Autodesk Inventor part; units mm, degrees
ref_plane "YZ Plane" through (0, 0, 0) normal (1, 0, 0) x (0, 1, 0)
ref_plane "XZ Plane" through (0, 0, 0) normal (0, 1, 0) x (-1, 0, 0)
ref_plane "XY Plane" through (0, 0, 0) normal (0, 0, 1) x (1, 0, 0)
sketch "Sketch1" plane through (0, 0, 0) normal (0, 1, 0) x (-1, 0, 0)
  line L0 (-88.0953, -35.095) -> (-78.6953, -35.095)
  line L1 (62.5047, 52.705) -> (71.9047, 52.705)
  line L2 (-88.0953, -35.095) -> (71.9047, -35.095)
  line L3 (71.9047, -35.095) -> (71.9047, 52.705)
  line L4 (71.9047, 52.705) -> (-88.0953, 52.705)
  line L5 (-88.0953, 52.705) -> (-88.0953, -35.095)
  circle A0 centre (-79.9551, -5.92) radius 2.7
  circle A1 centre (-79.9551, -5.92) radius 2.7
  circle A2 centre (-79.9551, 23.53) radius 2.7
  circle A3 centre (-79.9551, 23.53) radius 2.7
  circle A4 centre (-8.0953, 8.805) radius 2.7
  circle A5 centre (-8.0953, 8.805) radius 2.7
  circle A6 centre (63.7645, -5.92) radius 2.7
  circle A7 centre (63.7645, -5.92) radius 2.7
  circle A8 centre (63.7645, 23.53) radius 2.7
  circle A9 centre (63.7645, 23.53) radius 2.7
  line L6 (-88.0953, -35.095) -> (71.9047, -35.095)
  line L7 (71.9047, -35.095) -> (71.9047, 52.705)
  line L8 (71.9047, 52.705) -> (-88.0953, 52.705)
  line L9 (-88.0953, 52.705) -> (-88.0953, -35.095)
  point P0 (0, 0)
  point P1 (-83.0953, -33.095)
extrude "Extrusion1" add sketch "Sketch1" along normal blind 3
sketch "Sketch2" plane through (0, 3, 0) normal (0, 1, 0) x (1, 0, 0)
  circle A0 centre (8.0953, -8.805) radius 2.7
  line L0 (8.0953, -8.805) -> (8.0953, -52.705)
  line L1 (-71.9047, -52.705) -> (88.0953, -52.705)
  line L2 (8.0953, -8.805) -> (8.0953, 35.095)
  line L3 (88.0953, 35.095) -> (-71.9047, 35.095)
  line L4 (8.0953, -8.805) -> (-35.8047, -52.705)
  line L5 (8.0953, -8.805) -> (70.1793, -8.805) construction
  line L6 (8.0953, -8.805) -> (51.9953, -52.705)
  line L7 (8.0953, -8.805) -> (70.1793, -8.805) construction
  line L8 (8.0953, -8.805) -> (-18.3888, -8.805)
  line L9 (8.0953, -8.805) -> (-35.8047, 35.095)
  line L10 (8.0953, -8.805) -> (51.9953, 35.095)
  line L11 (-35.8047, -52.705) -> (51.9953, -52.705)
  line L12 (51.9953, -52.705) -> (51.9953, 35.095)
  line L13 (51.9953, 35.095) -> (-35.8047, 35.095)
  line L14 (-35.8047, 35.095) -> (-35.8047, -52.705)
  line L15 (8.0953, -8.805) -> (8.0953, -28.805)
  line L16 (8.0953, -28.805) -> (8.0953, 11.195)
  line L17 (8.0953, 11.195) -> (-15.8047, 35.095)
  line L18 (8.0953, -28.805) -> (-15.8047, -52.705)
  line L19 (8.0953, -28.805) -> (31.9953, -52.705)
  line L20 (8.0953, 11.195) -> (31.9953, 35.095)
  point P0 (0, 0)
  dimension "d2" = 135
  dimension "d3" = 45
  dimension "d4" = 20
  dimension "d5" = 40
extrude "Extrusion2" cut sketch "Sketch2" against normal blind 3 contours L17 L3 L2 | L2 L3 L20 | L19 L1 L0 | L0 L1 L18
sketch "Sketch3" plane through (0, 3, 0) normal (0, 1, 0) x (1, 0, 0)
  line L0 (-71.9047, 35.095) -> (-71.9047, -52.705)
  line L1 (-71.9047, -8.805) -> (-34.7047, -8.805)
  circle A0 centre (-34.7047, -8.805) radius 10
  point P0 (0, 0)
  dimension "d8" = 37.2
  dimension "d9" = 20
extrude "Extrusion3" cut sketch "Sketch3" against normal blind 3
sketch "Sketch4" plane through (0, 3, 0) normal (0, 1, 0) x (1, 0, 0)
  point P0 (0, 0)
sketch "Sketch5" plane through (0, 3, 0) normal (0, 1, 0) x (1, 0, 0)
  line L0 (-71.9047, 35.095) -> (-71.9047, -52.705)
  line L1 (88.0953, -52.705) -> (88.0953, 35.095)
  line L2 (-71.9047, -52.705) -> (88.0953, -52.705)
  line L3 (8.0953, -52.705) -> (8.0953, 35.095)
  circle A0 centre (-34.7047, -8.805) radius 10
  circle A1 centre (-34.7047, -8.805) radius 10
  circle A2 centre (50.8953, -8.805) radius 10
  point P0 (0, 0)
extrude "Extrusion4" cut sketch "Sketch5" against normal blind 3 contours A2
sketch "Sketch6" plane through (0, 3, 0) normal (0, 1, 0) x (1, 0, 0)
  line L0 (-48.5025, 4.8798) -> (-18.5618, 4.8798)
  line L1 (-18.5618, 4.8798) -> (-18.5618, -20.2546)
  line L2 (-18.5618, -20.2546) -> (-48.5025, -20.2546)
  line L3 (-48.5025, -20.2546) -> (-48.5025, 4.8798)
  point P0 (0, 0)
extrude "Extrusion5" add sketch "Sketch6" against normal up to surface (3 mm away)
sketch "Sketch7" plane through (0, 3, 0) normal (0, 1, 0) x (1, 0, 0)
  line L0 (-15.8047, 35.095) -> (-71.9047, 35.095)
  line L1 (-71.9047, 35.095) -> (8.0953, 35.095)
  line L2 (8.0953, 35.095) -> (8.0953, -52.705)
  line L3 (8.0953, -52.705) -> (-71.9047, -52.705)
  line L4 (-71.9047, -52.705) -> (-71.9047, 35.095)
  line L5 (-71.9047, -8.805) -> (8.0953, -8.805)
  line L6 (-31.9047, -8.805) -> (-52.4047, -8.805)
  line L7 (-52.4047, -8.805) -> (-11.4047, -8.805)
  line L8 (-52.4047, -8.805) -> (-11.4047, -8.805)
  line L9 (-11.4047, -8.805) -> (-11.4047, 25.695)
  line L10 (-11.4047, 25.695) -> (-52.4047, 25.695)
  line L11 (-52.4047, 25.695) -> (-52.4047, -8.805)
  line L12 (-52.4047, 25.695) -> (-11.4047, 25.695)
  line L13 (-11.4047, 25.695) -> (-11.4047, -43.305)
  line L14 (-11.4047, -43.305) -> (-52.4047, -43.305)
  line L15 (-52.4047, -43.305) -> (-52.4047, 25.695)
  line L16 (-31.9047, -8.805) -> (-31.9047, -5.9886)
  line L17 (-31.9047, -5.9886) -> (-50.3547, -5.9886)
  line L18 (-50.3547, -5.9886) -> (-13.4547, -5.9886)
  line L19 (-50.4047, 23.695) -> (-13.4047, 23.695)
  line L20 (-13.4047, 23.695) -> (-13.4047, -41.305)
  line L21 (-13.4047, -41.305) -> (-50.4047, -41.305)
  line L22 (-50.4047, -41.305) -> (-50.4047, 23.695)
  point P0 (0, 0)
  dimension "d16" = 20.5
  dimension "d17" = 41
  dimension "d18" = 34.5
  dimension "d19" = 69
  dimension "d20" = 18.45
  dimension "d21" = 36.9
  dimension "d22" = 2
extrude "Extrusion6" add sketch "Sketch7" along normal blind 18.5 contours L11 L10 L9 L5 L20 L19 L22 | L5 L22 L21 L20 L13 L14 L15
properties part number "SCHOOL PROJECT TOP"
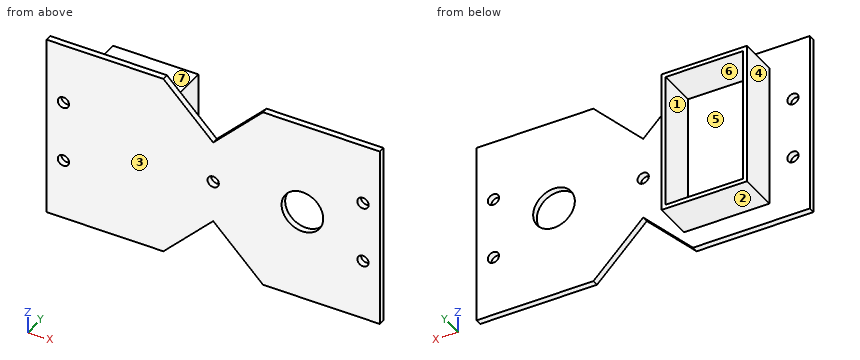
Work out the finished part from the listing and answer in its coordinate system (mm). Face numbers are marked on the shaded views. A direction names the side the tool comes from. Round coordinates to 2 decimals unless told otherwise and drop trailing zeros. Loops run counter-clockwise (first coordinate to the right, second up) from the corner with the lowest first, then second, coordinate; pieces in that order, holes last.
(1) Find the intervals of material crossed by L1, parallel to X at y = 8.5, z = 27.5; L2, parallel to Z at x = -15, y = 8.5 (3 decimals); L3, parallel to Y at x = -41.5, z = 6, in increasing order.
Computed values:
L1: x = -52.4 to -50.4, -13.4 to -11.4
L2: z = -25.695 to -23.695, 41.305 to 43.305
L3: y = 0 to 3
(2) The mould has two halves that part along X. Classify the marked faces 4, 5, 6 and 7: pulls with the +X half, pulls with the -X half, needs draft (parallel to the pull), parting line crosses it, or undercut.
Computed values:
face 4: pulls with the -X half
face 5: undercut
face 6: undercut
face 7: needs draft
(3) The part is cut by section B-B, the plane y = 8.75. Give the vertices of the cut face in (x, z) (3 decimals), and give its area (3 significant figures).
Computed values:
outline: (-52.405, -25.695) - (-11.405, -25.695) - (-11.405, 43.305) - (-52.405, 43.305) - close; hole (-50.405, -23.695) - (-13.405, -23.695) - (-13.405, 41.305) - (-50.405, 41.305) - close
area: 424 mm2
(4) The part is cut by section D-D, the plane x = 75. Give the vertices of the cut face in (y, z) (3 decimals).
Computed values:
outline: (0, -35.095) - (3, -35.095) - (3, 52.705) - (0, 52.705) - close
(5) For the marked faces 1, 2 and 3, determine the directions among +Z, -Z, +X, -X, +Y, -Y from which every point of the face is accessible in a straight line to the end or side of a thin tool.
Computed values:
face 1: +Y
face 2: -Z, +X, -X, +Y
face 3: +Z, -Z, +X, -X, -Y
(6) Each of these flat-tipped pins is pushed along its axis until it touches: P1, Ø9, axis at x = -34, y = 15, coming from the +Z side (3 decimals); P2, Ø4, axis at y = 13.5, z = 1.5, coming from the -X side; P3, Ø5, axis at x = -3, z = 7.5, coming from the +Y side. Where does it stop, or does it pass through?
Computed values:
P1: stops at z = 43.305
P2: stops at x = -52.4
P3: stops at y = 3
(7) The part is cut by section C-C, the plane z = 35. Give the vertices of the cut face in (x, y), and give its area (3 significant figures).
Computed values:
outline: (-71.9, 0) - (1.9, 0) - (1.9, 3) - (-11.4, 3) - (-11.4, 21.5) - (-13.4, 21.5) - (-13.4, 3) - (-50.4, 3) - (-50.4, 21.5) - (-52.4, 21.5) - (-52.4, 3) - (-71.9, 3) - close; (14.29, 0) - (88.1, 0) - (88.1, 3) - (14.29, 3) - close
area: 517 mm2
(8) The part is cut by section A-A, the plane z = -5.92. Give the vertices of the cut face in (x, y).
Computed values:
outline: (-71.9, 0) - (-66.46, 0) - (-66.46, 3) - (-71.9, 3) - close; (-61.06, 0) - (77.26, 0) - (77.26, 3) - (-11.4, 3) - (-11.4, 21.5) - (-13.4, 21.5) - (-13.4, 3) - (-50.4, 3) - (-50.4, 21.5) - (-52.4, 21.5) - (-52.4, 3) - (-61.06, 3) - close; (82.66, 0) - (88.1, 0) - (88.1, 3) - (82.66, 3) - close
